from build123d import *

# Parameters (mm, degrees)
SKETCH2_R           = 17.5
BOSS_EXTRUDE2_DEPTH = 29
FILLET2_R           = 1
SKETCH3_R           = 18.5
BOSS_EXTRUDE3_DEPTH = 29.5
SKETCH4_R           = 6
BOSS_EXTRUDE4_DEPTH = 6
FILLET6_R           = 0.2
SKETCH5_R           = 3
BOSS_EXTRUDE5_DEPTH = 3
BOSS_EXTRUDE6_DEPTH = 12


with BuildPart() as part:
    # Sketch2 → Boss-Extrude2 (new body)
    with BuildSketch(Plane.XY):
        Circle(SKETCH2_R)
    extrude(amount=BOSS_EXTRUDE2_DEPTH)

    # Fillet2
    fillet2_edges = [part.edges().sort_by_distance(p)[0] for p in [
        (-17.5, 0, 29),
    ]]
    fillet(fillet2_edges, radius=FILLET2_R)

    # Sketch3 → Boss-Extrude3 (add)
    with BuildSketch(Plane.XY.offset(29)):
        Circle(SKETCH3_R)
    extrude(amount=BOSS_EXTRUDE3_DEPTH)

    # Sketch4 → Boss-Extrude4 (add)
    with BuildSketch(Plane.XY.offset(58.5)):
        with Locations((0, 7)):
            Circle(SKETCH4_R)
    extrude(amount=BOSS_EXTRUDE4_DEPTH)

    # Fillet6
    fillet6_edges = [part.edges().sort_by_distance(p)[0] for p in [
        (-6, 7, 64.5),
    ]]
    fillet(fillet6_edges, radius=FILLET6_R)

    # Sketch5 → Boss-Extrude5 (add)
    with BuildSketch(Plane.XY.offset(64.5)):
        with Locations((0, 7)):
            Circle(SKETCH5_R)
    extrude(amount=BOSS_EXTRUDE5_DEPTH)

    # Sketch6 → Boss-Extrude6 (add)
    with BuildSketch(Plane.XY.offset(67.5)):
        with BuildLine():
            Line((-1.658312395, 9.5), (1.658312395, 9.5))
            ThreePointArc((1.658312395, 9.5), (0, 4), (-1.658312395, 9.5))
        make_face()
    extrude(amount=BOSS_EXTRUDE6_DEPTH)


solid = part.part
For this review, take the finished solid that the model builds, in its own axes (mm). A direction names the side the tool comes from. Round coordinates to 2 decimals unless told otherwise and drop trailing zeros. Loops run counter-clockwise (first coordinate to the right, second up) from the corner with the lowest first, then second, coordinate; pieces in that order, holes last. Notation, with made-up numbers: (24.25, 84) - (34.25, 84) arc R30 cw to (34.25, 116) - close; hole circle Ø4 at (4.5, 23.5). An arc over 180 degrees is marked (long way). Use one line per item in the form item = value.
1) We need section C-C on z = 57. Write out the cut boundary in (x, y).
Solutions:
outline = circle Ø37 at (0, 0)
2) Tool access review of faces 1 (the face through (-0.78, 12.95, 61.36)), 2 (the face through (-4.01, -18.06, 43.54)), 3 (the face through (-13.887, -10.648, 13.804)): name each direction out of +Z, -Z, +X, -X, +Y, -Y from which nothing blocks a thin tool from reaching the whole face with its end or side.
Solutions:
face_1 = +Z
face_2 = +Z, -Z
face_3 = -Z
3) Mouldability with a two-part tool opening along Z and no side actions: class faces 4 (the face through (-17, -3, 29)), 5 (the face through (0, 0, 0)), 6 (the face through (0, 0, 58.5)), 7 (the face through (0, 9.5, 73)) as pulls with the +Z half, pulls with the -Z half, needs draft (parallel to the pull), parting line crosses it, or undercut.
Solutions:
face_4 = undercut
face_5 = pulls with the -Z half
face_6 = pulls with the +Z half
face_7 = needs draft
4) We need section B-B on y = 0. Write out the cut boundary in (x, z), then the cut area to 3 significant figures.
Solutions:
outline = (-18.5, 29) - (-16.5, 29) arc R1 ccw to (-17.5, 28) - (-17.5, 0) - (17.5, 0) - (17.5, 28) arc R1 ccw to (16.5, 29) - (18.5, 29) - (18.5, 58.5) - (-18.5, 58.5) - close
area = 2,110 mm2
5) Clearance check with flat-ended pins moving along their axes: P1, Ø11, axis at x = -8, y = 0.5, coming from the +Z side; P2, Ø1.5, axis at x = -4, z = 39, coming from the -Y side; P3, Ø2, axis at x = -9.5, y = 8, coming from the -Z side; P4, Ø3.5, axis at x = -0.5, z = 74, coming from the +Y side. State where each tip first meets the part, or that it passes through.
Solutions:
P1 = 64.5
P2 = -18.21
P3 = 0
P4 = 9.5
6) We need section A-A on x = 0. Write out the cut boundary in (y, z).
Solutions:
outline = (-18.5, 29) - (-16.5, 29) arc R1 ccw to (-17.5, 28) - (-17.5, 0) - (17.5, 0) - (17.5, 28) arc R1 ccw to (16.5, 29) - (18.5, 29) - (18.5, 58.5) - (13, 58.5) - (13, 64.3) arc R0.2 ccw to (12.8, 64.5) - (10, 64.5) - (10, 67.5) - (9.5, 67.5) - (9.5, 79.5) - (4, 79.5) - (4, 64.5) - (1.2, 64.5) arc R0.2 ccw to (1, 64.3) - (1, 58.5) - (-18.5, 58.5) - close
7) Wall thickness on probe 1 along Z at (x, y) = (3.5, -16); probe 2 along Z at (x, y) = (-5, 4); probe 3 along X at (y, z) = (0.5, 13): over which ranges is each line inside the solid? List them lowest first.
Solutions:
probe_1 = 0 to 58.5
probe_2 = 0 to 64.5
probe_3 = -17.49 to 17.49
